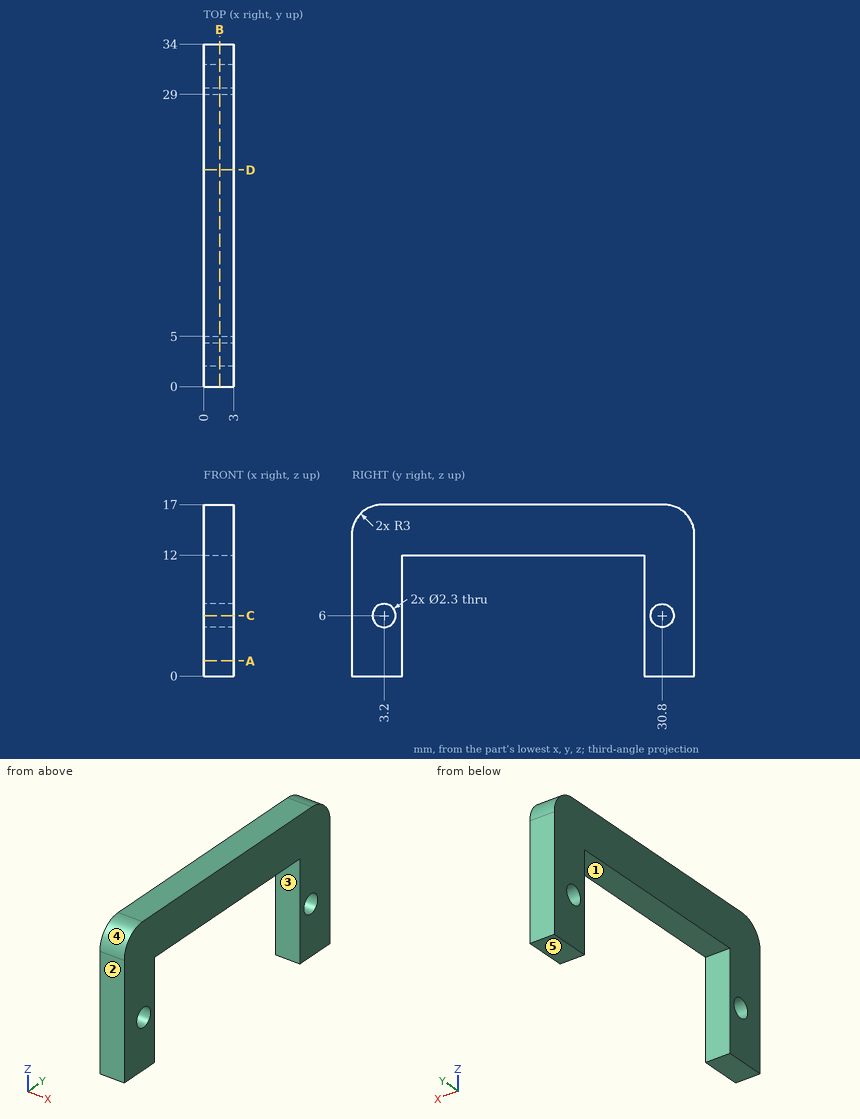
The drawing under review shows one solid part. Ordinate dimensions are in mm from its lowest x, y, z. A direction names the side the tool comes from. Round coordinates to 2 decimals unless told otherwise and drop trailing zeros. Order: outer loops, then holes, each group sorted by start corner. A loop starts at its lowest first (then second) coordinate and runs counter-clockwise, first axis right, second up. Notation, with made-up numbers: (-17.75, 63) -> (40.25, 63) arc R7 ccw to (40.25, 70) -> close; hole circle Ø4 at (27.25, 42.25). An arc over 180 degrees is marked (long way). Use a Markdown table: item, result.
Item 1: Take a section at C-C (z = 6). State the section outline as (x, y) points.
Resolved:
| item | result |
|---|---|
| outline | (0, 0) -> (3, 0) -> (3, 2.05) -> (0, 2.05) -> close; (0, 4.35) -> (3, 4.35) -> (3, 5) -> (0, 5) -> close; (0, 29) -> (3, 29) -> (3, 29.65) -> (0, 29.65) -> close; (0, 31.95) -> (3, 31.95) -> (3, 34) -> (0, 34) -> close |
Item 2: For pin 1 (10 mm diameter, centred on y = 13.5, z = 4, fed in from +X); pin 2 (0.9 mm diameter, centred on x = 1.5, y = 20, fed in from -Z), all flat-tipped, find the tip position at first contact; note any pin that passes through.
Resolved:
| item | result |
|---|---|
| pin 1 | passes through |
| pin 2 | stops at z = 12 |
Item 3: For line 1 along Y through (x, z) = (1.35, 11.5); line 2 along Z through (x, y) = (2.45, 3.2); line 3 along Z through (x, y) = (2.45, 23.5), list the stretches that pass through material, from the lowest coordinate up. Write a range as [from, to].
Resolved:
| item | result |
|---|---|
| line 1 | y = [0, 5], [29, 34] |
| line 2 | z = [0, 4.85], [7.15, 17] |
| line 3 | z = [12, 17] |
Item 4: Take a section at B-B (x = 1.6). State the section outline as (y, z) points.
Resolved:
| item | result |
|---|---|
| outline | (0, 0) -> (5, 0) -> (5, 12) -> (29, 12) -> (29, 0) -> (34, 0) -> (34, 14) arc R3 ccw to (31, 17) -> (3, 17) arc R3 ccw to (0, 14) -> close; hole circle Ø2.3 at (3.2, 6); hole circle Ø2.3 at (30.8, 6) |
Item 5: Machinability: for the marked faces 1 and 2, which of the approach directions +Z, -Z, +X, -X, +Y, -Y give a long, thin tool a straight path to every point of the face, cutting with its end or side? Answer none if there is none.
Resolved:
| item | result |
|---|---|
| face 1 | -Z, +X, -X |
| face 2 | +Z, -Z, +X, -X, -Y |
Item 6: Take a section at A-A (z = 1.5). State the section outline as (x, y) points.
Resolved:
| item | result |
|---|---|
| outline | (0, 0) -> (3, 0) -> (3, 5) -> (0, 5) -> close; (0, 29) -> (3, 29) -> (3, 34) -> (0, 34) -> close |
Item 7: Take a section at D-D (y = 21.5). State the section outline as (x, z) points, plus the area to 3 significant figures.
Resolved:
| item | result |
|---|---|
| outline | (0, 12) -> (3, 12) -> (3, 17) -> (0, 17) -> close |
| area | 15.0 mm² |
Item 8: Draft analysis for pull direction Y (two halves, no side actions). For the marked faces 3, 4 and 5, state which applies: +Y half, -Y half, draft (parallel to the pull), parting line (faces both ways), or undercut.
Resolved:
| item | result |
|---|---|
| face 3 | undercut |
| face 4 | -Y half |
| face 5 | draft |
